The figure shows three views and two pictorial views of one solid part (mm, origin at its lowest corner). Answer the questions. Give positions to 0.01 mm unless a question says otherwise; leave off trailing zeros. Loops run counter-clockwise (first coordinate to the right, second up) from the corner with the lowest first, then second, coordinate; pieces in that order, holes last. Notation, with made-up numbers: (87.5, -33) - (146.5, -33) arc R27 ccw to (146.5, -8) - close; hole circle Ø8 at (73, -24). An arc over 180 degrees is marked (long way). Use CSV: the item, a comma, the result in double quotes.
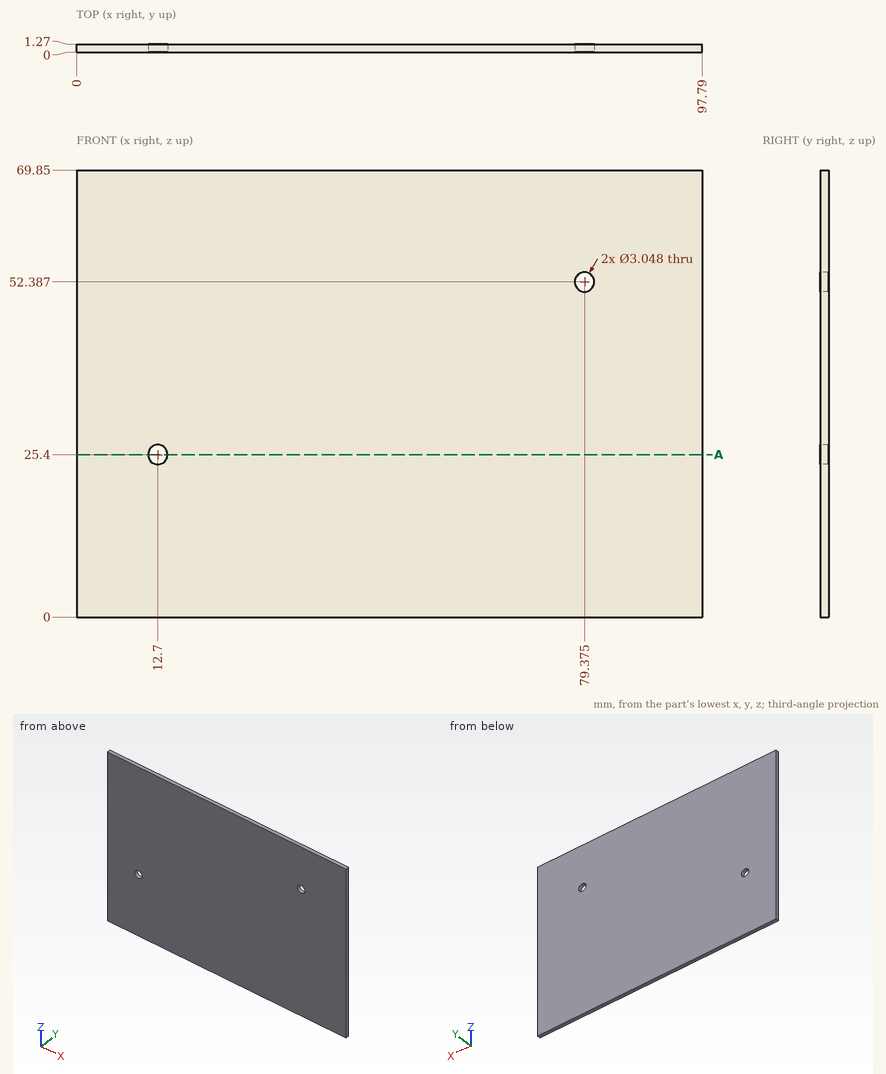
Item 1: A cutting plane is placed at A-A on z = 25.4. Determine the outline of the cut face in (x, y) (1 decimal).
Determined:
outline,"(0, 0) - (11.2, 0) - (11.2, 1.3) - (0, 1.3) - close; (14.2, 0) - (97.8, 0) - (97.8, 1.3) - (14.2, 1.3) - close"
Item 2: Given P1, Ø3.5, axis at x = 12.7, z = 25.4, coming from the +Y side, flat-ended and moving along its own axis, determine where the tip first touches the part or whether it passes through.
Determined:
P1,"stops at y = 1.27"
Item 3: Find the intervals of material crossed by line 1 (X direction, y = 0.3, z = 25.4) (1 decimal); line 2 (Z direction, x = 79.5, y = 0.8); line 3 (X direction, y = 1.05, z = 51.5) (1 decimal), in increasing order.
Determined:
line 1,"x = 0 to 11.2, 14.2 to 97.8"
line 2,"z = 0 to 50.87, 53.91 to 69.85"
line 3,"x = 0 to 78.1, 80.6 to 97.8"
